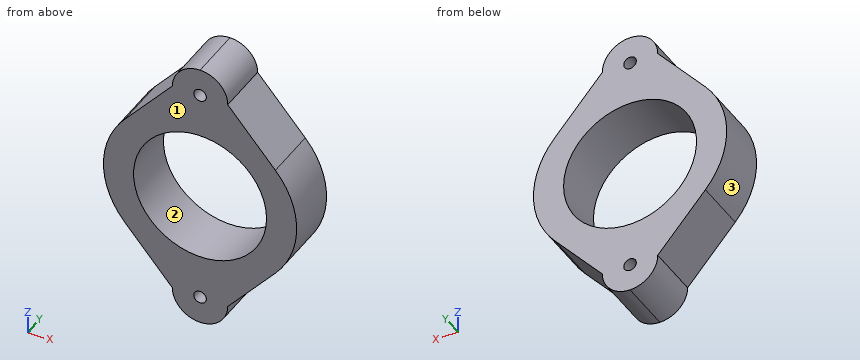
from build123d import *

# Parameters (mm, degrees)
F0_R     = 3.4
F0_R_2   = 36
F1_DEPTH = 29


with BuildPart() as f1:
    # F0 (on Front) → F1 (new body)
    with BuildSketch(Plane.XZ):
        with BuildLine():
            ThreePointArc((-99.807744, -65.08165), (-95.414346, -75.688252), (-84.807744, -80.08165))
            ThreePointArc((-84.807744, -80.08165), (-74.201142, -75.688252), (-69.807744, -65.08165))
            Line((-69.807744, -65.08165), (-44.015344, -35.68165))
            ThreePointArc((-44.015344, -35.68165), (-32.495199, -5.08165), (-44.015344, 25.51835))
            Line((-44.015344, 25.51835), (-69.807744, 54.91835))
            ThreePointArc((-69.807744, 54.91835), (-74.201142, 65.524952), (-84.807744, 69.91835))
            ThreePointArc((-84.807744, 69.91835), (-95.414346, 65.524952), (-99.807744, 54.91835))
            Line((-99.807744, 54.91835), (-125.607744, 25.51835))
            ThreePointArc((-125.607744, 25.51835), (-137.13044, -5.08165), (-125.607744, -35.68165))
            Line((-125.607744, -35.68165), (-99.807744, -65.08165))
        make_face()
        with Locations((-84.807744, -65.08165)):
            Circle(F0_R, mode=Mode.SUBTRACT)
        with Locations((-84.807744, -5.08165)):
            Circle(F0_R_2, mode=Mode.SUBTRACT)
        with Locations((-84.807744, 54.91835)):
            Circle(F0_R, mode=Mode.SUBTRACT)
    extrude(amount=F1_DEPTH)


solid = f1.part
Part model, mm, in its own coordinate system. Face numbers are marked on the shaded views. Coordinates: 2 decimals unless noted, no trailing zeros. Loops run counter-clockwise (first coordinate to the right, second up) from the corner with the lowest first, then second, coordinate; pieces in that order, holes last. Notation, with made-up numbers: M -3,70 L 34,70 A14 cw 34,92 Z; hole C -27,-20 d11. An arc over 180 degrees is marked long. Use a Markdown table: item, result. Add a question column.
Q1. Cut at A-A (z = -39.5). Write the cut outline in (x, y).
Q2. Cut at D-D (x = -47). Write the cut outline in (y, z).
Q3. Cut at C-C (y = -6). Write the cut outline in (x, z), and give its area (3 significant figures).
Q4. Mould opens along X. For the marked faces 1, 2 and 3 say: +X half, -X half, draft (parallel to the pull), parting line (faces both ways), or undercut.
Q5. Cut at B-B (x = -116.5). Write the cut outline in (y, z).
Q6. Probe L1, parallel to Z at x = -86, y = -9.5; L2, parallel to Z at x = -64.5, y = -3.5; L3, parallel to Z at x = -82.5, y = -12. List the from-to ranges inside material, lowest first.
Q7. Pin check, flat tips, straight feed: P1, Ø5, axis at y = -9, z = -25, coming from the +X side; P2, Ø6, axis at x = -123, y = -11.5, coming from the -Z side; P3, Ø1.5, axis at x = -101, y = -25.5, coming from the +Z side. Stop position of each tip, or through.
Worked out:
| question | item | result |
|---|---|---|
| 1 | outline | M -122.26,-29 L -95.36,-29 L -95.36,0 L -122.26,0 Z; M -74.25,-29 L -47.37,-29 L -47.37,0 L -74.25,0 Z |
| 2 | outline | M -29,-39.08 L 0,-39.08 L 0,28.92 L -29,28.92 Z |
| 3 | outline | M -125.61,-35.68 L -99.81,-65.08 A15 ccw -84.81,-80.08 A15 ccw -69.81,-65.08 L -44.02,-35.68 A46.4 ccw -44.02,25.52 L -69.81,54.92 A15 ccw -84.81,69.92 A15 ccw -99.81,54.92 L -125.61,25.52 A46.39 ccw Z; hole C -84.81,-5.08 d72; hole C -84.81,-65.08 d6.8; hole C -84.81,54.92 d6.8 |
| 3 | area | 5,800 mm2 |
| 4 | face 1 | draft |
| 4 | face 2 | undercut |
| 4 | face 3 | -X half |
| 5 | outline | M -29,-46.06 L 0,-46.06 L 0,-22.16 L -29,-22.16 Z; M -29,11.99 L 0,11.99 L 0,35.9 L -29,35.9 Z |
| 6 | L1 | z = -80.03 to -68.27, -61.9 to -41.06, 30.9 to 51.73, 58.1 to 69.87 |
| 6 | L2 | z = -59.03 to -34.81, 24.64 to 48.87 |
| 6 | L3 | z = -79.9 to -67.58, -62.58 to -41.01, 30.84 to 52.42, 57.42 to 69.74 |
| 7 | P1 | stops at x = -35.89 |
| 7 | P2 | stops at z = -42.07 |
| 7 | P3 | stops at z = 54.41 |
